```python
from build123d import *

# Parameters (mm, degrees)
SKETCH_3_R          = 3.00000508
EXTRUDE_1_DEPTH     = 1.6
SKETCH_4_W          = 1
SKETCH_4_H          = 1
EXTRUDE_2_DEPTH     = 1
SKETCH_5_W          = 3.8001016
SKETCH_5_H          = 3.8001016
EXTRUDE_3_DEPTH     = 1.5
SKETCH_6_R          = 1.9000508
EXTRUDE_4_DEPTH     = 4
SKETCH_7_R          = 1.615152196
CUT_EXTRUDE_1_DEPTH = 4
SKETCH_8_R          = 0.601590178
EXTRUDE_5_DEPTH     = 3
SKETCH_9_R          = 0.306574413
CUT_EXTRUDE_2_DEPTH = 3
SKETCH_10_W         = 0.228686602
SKETCH_10_H         = 1.655690995
CUT_EXTRUDE_3_DEPTH = 3


with BuildPart() as part:
    # 草图3 → 凸台-拉伸1 (new body)
    with BuildSketch(Plane.XY):
        with Locations((3.00000508, 3.00000508)):
            Circle(SKETCH_3_R)
    extrude(amount=EXTRUDE_1_DEPTH)

    # 草图4 → 凸台-拉伸2 (add)
    with BuildSketch(Plane(origin=(0, 0, 0), x_dir=(-1, 0, 0), z_dir=(0, 0, -1))):
        with Locations((-1.59995428, 1.59995428)):
            Rectangle(SKETCH_4_W, SKETCH_4_H)
        with Locations((-1.59995428, 4.40005588)):
            Rectangle(SKETCH_4_W, SKETCH_4_H)
        with Locations((-4.40005588, 4.40005588)):
            Rectangle(SKETCH_4_W, SKETCH_4_H)
        with Locations((-4.40005588, 1.59995428)):
            Rectangle(SKETCH_4_W, SKETCH_4_H)
    extrude(amount=EXTRUDE_2_DEPTH)

    # 草图5 → 凸台-拉伸3 (add)
    with BuildSketch(Plane(origin=(0, 0, -1), x_dir=(-1, 0, 0), z_dir=(0, 0, -1))):
        with Locations((-3.00000508, 3.00000508)):
            Rectangle(SKETCH_5_W, SKETCH_5_H)
    extrude(amount=EXTRUDE_3_DEPTH)

    # 草图6 → 凸台-拉伸4 (add)
    with BuildSketch(Plane(origin=(0, 0, -2.5), x_dir=(-1, 0, 0), z_dir=(0, 0, -1))):
        with Locations((-3.00000508, 3.00000508)):
            Circle(SKETCH_6_R)
    extrude(amount=EXTRUDE_4_DEPTH)

    # 草图7 → 切除-拉伸1 (cut)
    with BuildSketch(Plane(origin=(0, 0, -6.5), x_dir=(-1, 0, 0), z_dir=(0, 0, -1))):
        with Locations((-3.00000508, 3.00000508)):
            Circle(SKETCH_7_R)
    extrude(amount=-CUT_EXTRUDE_1_DEPTH, mode=Mode.SUBTRACT)

    # 草图8 → 凸台-拉伸5 (add)
    with BuildSketch(Plane(origin=(0, 0, -2.5), x_dir=(-1, 0, 0), z_dir=(0, 0, -1))):
        with Locations((-3.00000508, 3.00000508)):
            Circle(SKETCH_8_R)
    extrude(amount=EXTRUDE_5_DEPTH)

    # 草图9 → 切除-拉伸2 (cut)
    with BuildSketch(Plane(origin=(0, 0, -5.5), x_dir=(-1, 0, 0), z_dir=(0, 0, -1))):
        with Locations((-3.00000508, 3.00000508)):
            Circle(SKETCH_9_R)
    extrude(amount=-CUT_EXTRUDE_2_DEPTH, mode=Mode.SUBTRACT)

    # 草图10 → 切除-拉伸3 (cut)
    with BuildSketch(Plane(origin=(0, 0, -5.5), x_dir=(-1, 0, 0), z_dir=(0, 0, -1))):
        with Locations((-2.999022369, 2.996212045)):
            Rectangle(SKETCH_10_W, SKETCH_10_H)
    extrude(amount=-CUT_EXTRUDE_3_DEPTH, mode=Mode.SUBTRACT)


solid = part.part
```
Input: part model. Units: mm. Frame: model coordinates. A direction names the side the tool comes from. Coordinates: 2 decimals unless noted, no trailing zeros. Loops run counter-clockwise (first coordinate to the right, second up) from the corner with the lowest first, then second, coordinate; pieces in that order, holes last.
Q1. Line query: line 1 along Y through (x, z) = (3, -5); line 2 along Y through (x, z) = (4, -0.5); line 3 along Z through (x, y) = (4, 3.5). Output: solid intervals per line, ascending.
Results are:
line 1: y = 1.1 to 1.38, 4.62 to 4.9
line 2: y = 1.1 to 2.1, 3.9 to 4.9
line 3: z = -2.5 to -1, 0 to 1.6
Q2. Contact query for flat-ended pins moving along their axis: pin 1 (3 mm diameter, centred on y = 2.5, z = -1, fed in from -X); pin 2 (0.5 mm diameter, centred on x = 3.5, y = 3, fed in from -Z); pin 3 (3 mm diameter, centred on y = 4.5, z = -3.5, fed in from +X); pin 4 (2 mm diameter, centred on x = 0.5, z = 0, fed in from +Y). Output: stop coordinate, or through.
Results are:
pin 1: stops at x = 0
pin 2: stops at z = -5.5
pin 3: stops at x = 4.9
pin 4: stops at y = 5.6
Q3. Set-up query: faces 1 (the flat face through (3.9, 1.6, -0.5)), 2 (the flat face through (4.5, 4.4, -2.5)), 3 (the flat face through (4.4, 3.9, -0.5)). Return all of +Z, -Z, +X, -X, +Y, -Y with unobstructed straight access to the full face (end or side cutting, diameter ignored); none if empty.
Results are:
face 1: +Y, -Y
face 2: -Z, +X, +Y
face 3: +X, -X
Q4. Section A-A, the plane z = -5. Return the cut outline in (x, y), and give its area (3 significant figures).
Results are:
outline: circle Ø3.8 at (3, 3); (2.88, 2.41) - (2.88, 2.72) arc R0.31 cw to (2.88, 3.28) - (2.88, 3.59) arc R0.6 ccw to start; (3.11, 2.41) arc R0.6 ccw to (3.11, 3.59) - (3.11, 3.28) arc R0.31 cw to (3.11, 2.72) - close; hole circle Ø3.23 at (3, 3)
area: 3.85 mm2
Q5. Mould query, pull axis X, two halves, no side actions, for faces 4 (the cylindrical face through (4.4, 4.284, -4.472)), 5 (the flat face through (2.1, 1.6, -0.5)), 6 (the flat face through (1.6, 3.9, -0.5)). Classes: +X half, -X half, draft (parallel to the pull), parting line (faces both ways), or undercut.
Results are:
face 4: parting line
face 5: undercut
face 6: draft
Q6. Section D-D, the plane x = 1.5. Return the cut outline in (y, z).
Results are:
outline: (0.4, 0) - (1.1, 0) - (1.1, -2.5) - (1.83, -2.5) - (1.83, -6.5) - (2.4, -6.5) - (2.4, -2.5) - (3.6, -2.5) - (3.6, -6.5) - (4.17, -6.5) - (4.17, -2.5) - (4.9, -2.5) - (4.9, 0) - (5.6, 0) - (5.6, 1.6) - (0.4, 1.6) - close; hole (2.1, -1) - (3.9, -1) - (3.9, 0) - (2.1, 0) - close
Q7. Section B-B, the plane x = 3.75. Return the cut outline in (y, z), and give its area (3 significant figures).
Results are:
outline: (0.1, 0) - (5.9, 0) - (5.9, 1.6) - (0.1, 1.6) - close; (1.1, -2.5) - (1.25, -2.5) - (1.25, -6.5) - (1.57, -6.5) - (1.57, -2.5) - (4.43, -2.5) - (4.43, -6.5) - (4.75, -6.5) - (4.75, -2.5) - (4.9, -2.5) - (4.9, -1) - (1.1, -1) - close
area: 17.5 mm2
